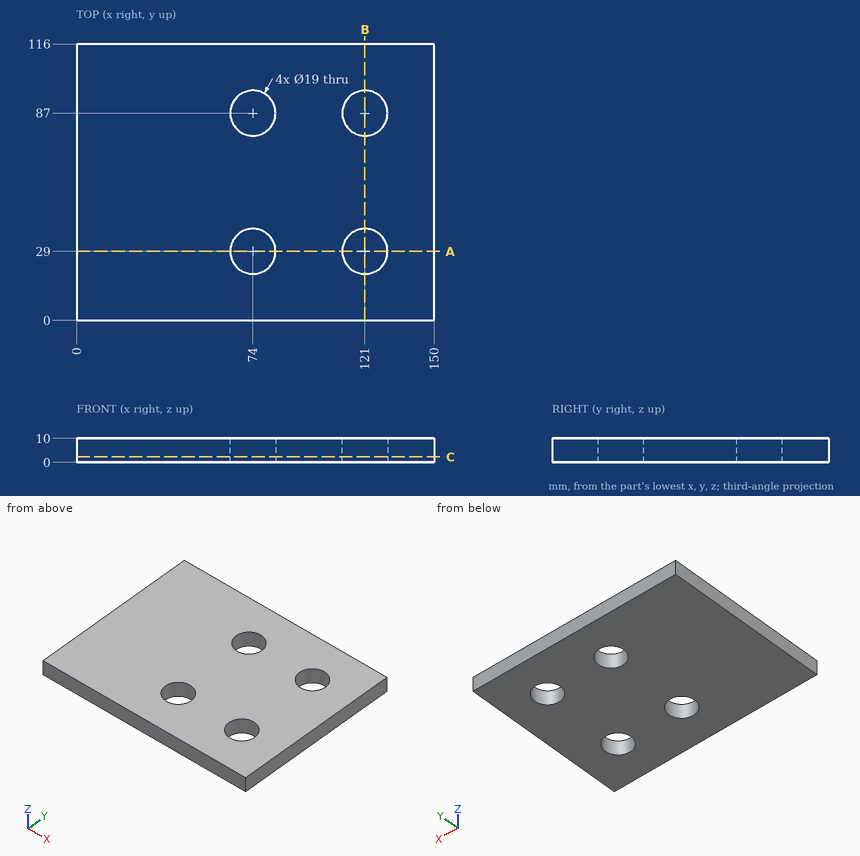
Source: three-view drawing plus pictorial views. Frame: mm from the lowest corner of the part. Round coordinates to 2 decimals unless told otherwise and drop trailing zeros. Loops run counter-clockwise (first coordinate to the right, second up) from the corner with the lowest first, then second, coordinate; pieces in that order, holes last. Notation, with made-up numbers: M -1.5,-38.75 L 53.5,-38.75 A14 ccw 53.5,-17.75 Z; hole C 26,7 d1. An arc over 180 degrees is marked long. Put each result on its own line as item: value. Start each with the question number.
(1) Material intervals for line 1 along Y through (x, z) = (121, 6.25); line 2 along Y through (x, z) = (114.5, 3); line 3 along X through (y, z) = (91.5, 5), sorted ascending. Write a range as [from, to].
(2) Section query C-C (z = 2.25). Return loops of the section in (x, y).
(3) Section query B-B (x = 121). Return loops of the section in (y, z).
(4) Section query A-A (y = 29). Return loops of the section in (x, z), then the cut area to 3 significant figures.
(5) Contact query for a flat-ended pin moving along its axis: pin 1 Ø11.5 at (x, y) = (74, 87) entering from +Z. Output: stop coordinate, or through.
Findings below:
1. line 1: y = [0, 19.5], [38.5, 77.5], [96.5, 116]
1. line 2: y = [0, 22.07], [35.93, 80.07], [93.93, 116]
1. line 3: x = [0, 65.63], [82.37, 112.63], [129.37, 150]
2. outline: M 0,0 L 150,0 L 150,116 L 0,116 Z; hole C 74,29 d19; hole C 74,87 d19; hole C 121,29 d19; hole C 121,87 d19
3. outline: M 0,0 L 19.5,0 L 19.5,10 L 0,10 Z; M 38.5,0 L 77.5,0 L 77.5,10 L 38.5,10 Z; M 96.5,0 L 116,0 L 116,10 L 96.5,10 Z
4. outline: M 0,0 L 64.5,0 L 64.5,10 L 0,10 Z; M 83.5,0 L 111.5,0 L 111.5,10 L 83.5,10 Z; M 130.5,0 L 150,0 L 150,10 L 130.5,10 Z
4. area: 1,120 mm2
5. pin 1: passes through
